Geometry check sheet. Reference: the model listing, model coordinates, mm. Face numbers are marked on the shaded views. A direction names the side the tool comes from. Round coordinates to 2 decimals unless told otherwise and drop trailing zeros. Loops run counter-clockwise (first coordinate to the right, second up) from the corner with the lowest first, then second, coordinate; pieces in that order, holes last.
```python
from build123d import *

# Parameters (mm, degrees)
SKETCH1_W                = 22.606
SKETCH1_H                = 11.938
BOSS_EXTRUDE1_DEPTH      = 25.4
SKETCH2_R                = 2.224672202
BOSS_EXTRUDE2_DEPTH      = 4.572
SKETCH3_R                = 4.279679958
BOSS_EXTRUDE3_DEPTH      = 1.27
BOSS_EXTRUDE4_DEPTH      = 7.62
BOSS_EXTRUDE4_DEPTH_BACK = 30.48
SKETCH4_W                = 11.938
SKETCH4_H                = 2.54


with BuildPart() as part:
    # Sketch1 → Boss-Extrude1 (new body)
    with BuildSketch(Plane(origin=(0, 0, 0), x_dir=(1, 0, 0), z_dir=(0, 1, 0))):
        with Locations((11.303, 5.969)):
            Rectangle(SKETCH1_W, SKETCH1_H)
    extrude(amount=BOSS_EXTRUDE1_DEPTH)

    # Sketch2 → Boss-Extrude2 (add)
    with BuildSketch(Plane(origin=(0, 25.4, 0), x_dir=(1, 0, 0), z_dir=(0, 1, 0))):
        with Locations(Location((4.707032939, 5.969, 0), (0, 0, 90))):
            Circle(SKETCH2_R)
    extrude(amount=BOSS_EXTRUDE2_DEPTH)

    # Sketch3 → Boss-Extrude3 (add)
    with BuildSketch(Plane(origin=(0, 25.4, 0), x_dir=(1, 0, 0), z_dir=(0, 1, 0))):
        with Locations(Location((4.707032939, 5.969, 0), (0, 0, 90))):
            Circle(SKETCH3_R)
    extrude(amount=BOSS_EXTRUDE3_DEPTH)

    # Sketch4 → Boss-Extrude4 (add, two sides: drawn at the far end of the back side and taken through both)
    with BuildSketch(Plane(origin=(22.606, 0, 0), x_dir=(0, 0, -1), z_dir=(1, 0, 0)).offset(-BOSS_EXTRUDE4_DEPTH_BACK)):
        with Locations((5.969, 18.034)):
            Rectangle(SKETCH4_W, SKETCH4_H)
    extrude(amount=BOSS_EXTRUDE4_DEPTH + BOSS_EXTRUDE4_DEPTH_BACK)


solid = part.part
```
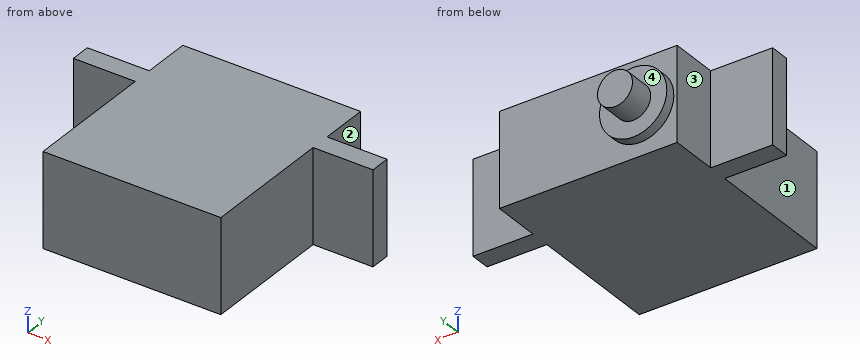
1) Gauge pin test, flat ends, axial feed: pin 1 (1.5 mm diameter, centred on y = 25.5, z = -5.5, fed in from +X); pin 2 (6 mm diameter, centred on y = 4.5, z = -2, fed in from -X); pin 3 (6.5 mm diameter, centred on x = -2.5, z = -6, fed in from +Y). Record the tip position at first contact, or that the pin passes through.
Report:
pin 1: stops at x = 22.61
pin 2: stops at x = 0
pin 3: stops at y = 26.67
2) Sectioned sample at D-D, the plane z = -5.25. Record the cut outline in (x, y), then the cut area to 3 significant figures.
Report:
outline: (-7.87, 16.76) - (0, 16.76) - (0, 0) - (22.61, 0) - (22.61, 16.76) - (30.23, 16.76) - (30.23, 19.3) - (22.61, 19.3) - (22.61, 25.4) - (8.93, 25.4) - (8.93, 26.67) - (6.81, 26.67) - (6.81, 29.97) - (2.6, 29.97) - (2.6, 26.67) - (0.49, 26.67) - (0.49, 25.4) - (0, 25.4) - (0, 19.3) - (-7.87, 19.3) - close
area: 638 mm2
3) Sectioned sample at A-A, the plane z = -10.75. Record the cut outline in (x, y).
Report:
outline: (-7.87, 16.76) - (0, 16.76) - (0, 0) - (22.61, 0) - (22.61, 16.76) - (30.23, 16.76) - (30.23, 19.3) - (22.61, 19.3) - (22.61, 25.4) - (0, 25.4) - (0, 19.3) - (-7.87, 19.3) - close
4) Scan lines: line 1 along Y through (x, z) = (19, -9); line 2 along X through (y, z) = (9, -1.5); line 3 along Y through (x, z) = (27, -1). Record each from-to range of solid material in increasing order.
Report:
line 1: y = 0 to 25.4
line 2: x = 0 to 22.61
line 3: y = 16.76 to 19.3
5) Sectioned sample at B-B, the plane x = 5.5. Record the cut outline in (y, z), then the cut area to 3 significant figures.
Report:
outline: (0, -11.94) - (25.4, -11.94) - (25.4, -10.17) - (26.67, -10.17) - (26.67, -8.05) - (29.97, -8.05) - (29.97, -3.89) - (26.67, -3.89) - (26.67, -1.76) - (25.4, -1.76) - (25.4, 0) - (0, 0) - close
area: 328 mm2
6) Access from +Z, -Z, +X, -X, +Y, -Y to the whole of each face (thin tool, end or side, straight path). Record for the marked faces 1, 2, 3 and 4.
Report:
face 1: +Z, -Z, -X, -Y
face 2: +Z, -Z, +X, +Y
face 3: +Z, -Z, -X, +Y
face 4: +Y
7) Sectioned sample at C-C, the plane y = 23.25. Record the cut outline in (x, z), then the cut area to 3 significant figures.
Report:
outline: (0, -11.94) - (22.61, -11.94) - (22.61, 0) - (0, 0) - close
area: 270 mm2
